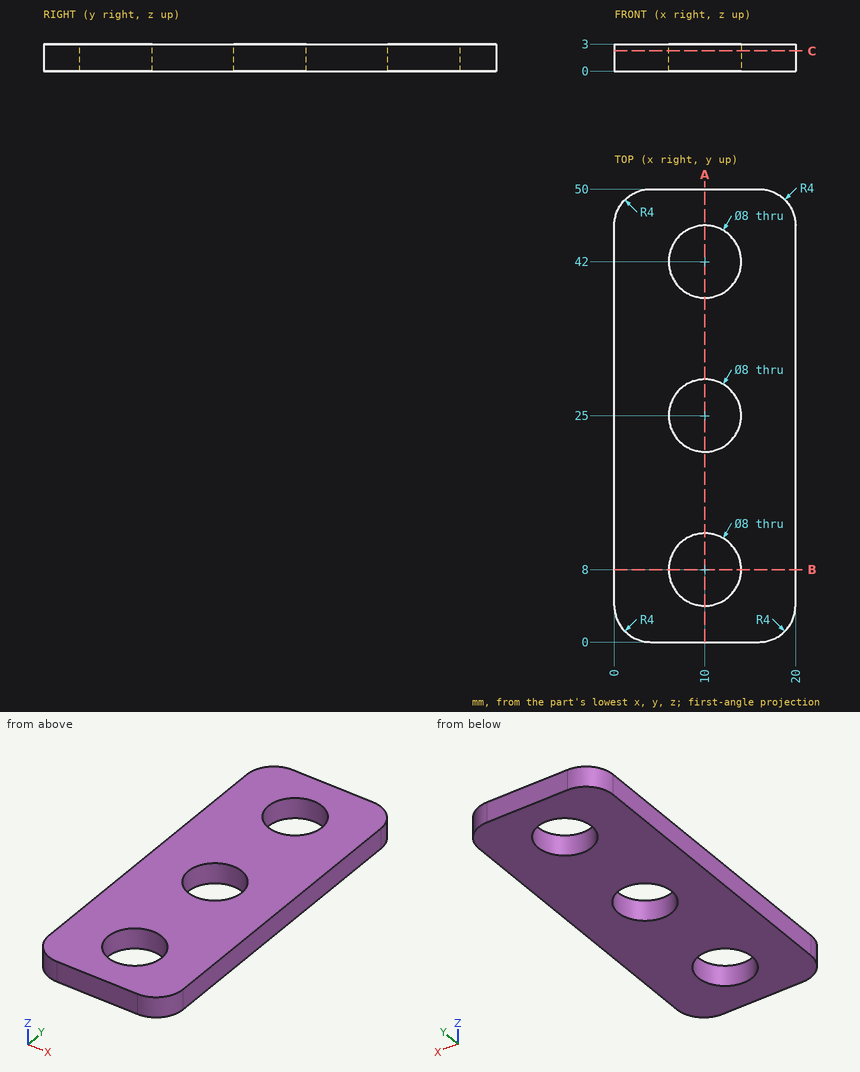
Print and shaded views of the part. All mm, measured from the part's lowest x, y and z. Give positions to 0.01 mm unless a question says otherwise; leave off trailing zeros. Loops run counter-clockwise (first coordinate to the right, second up) from the corner with the lowest first, then second, coordinate; pieces in that order, holes last. Notation, with made-up numbers: (-32.5, 33) -> (-10.5, 33) arc R31 cw to (-10.5, 61) -> close; hole circle Ø8 at (-37.75, 38). An arc over 180 degrees is marked (long way). One line per question, with ' | ' between items. Start each with the question number.
1) Cut at C-C (z = 2.25). Give the cut face in (x, y).
2) Probe L1, parallel to Y at x = 10, z = 2.2; L2, parallel to Y at x = 7.75, z = 2.1; L3, parallel to X at y = 10, z = 1. List the from-to ranges inside material, lowest first.
3) Cut at B-B (y = 8). Give the cut face in (x, z), plus the area to 3 significant figures.
4) Cut at A-A (x = 10). Give the cut face in (y, z).
Return value:
1) outline: (0, 4) arc R4 ccw to (4, 0) -> (16, 0) arc R4 ccw to (20, 4) -> (20, 46) arc R4 ccw to (16, 50) -> (4, 50) arc R4 ccw to (0, 46) -> close; hole circle Ø8 at (10, 8); hole circle Ø8 at (10, 25); hole circle Ø8 at (10, 42)
2) L1: 0 to 4, 12 to 21, 29 to 38, 46 to 50 | L2: 0 to 4.69, 11.31 to 21.69, 28.31 to 38.69, 45.31 to 50 | L3: 0 to 6.54, 13.46 to 20
3) outline: (0, 0) -> (6, 0) -> (6, 3) -> (0, 3) -> close; (14, 0) -> (20, 0) -> (20, 3) -> (14, 3) -> close | area: 36.0 mm^2
4) outline: (0, 0) -> (4, 0) -> (4, 3) -> (0, 3) -> close; (12, 0) -> (21, 0) -> (21, 3) -> (12, 3) -> close; (29, 0) -> (38, 0) -> (38, 3) -> (29, 3) -> close; (46, 0) -> (50, 0) -> (50, 3) -> (46, 3) -> close
